Source: CAD feature listing. Evaluate the final solid. Frame: model axes, mm. A direction names the side the tool comes from. Give positions to 0.01 mm unless a question says otherwise; leave off trailing zeros. Write each loop counter-clockwise with the first axis right and the second up, starting at its lowest first coordinate (ties: lowest second). Pieces come first, ordered by that corner, then holes. Notation, with made-up numbers: (-22, 20) -> (9, 20) arc R18 cw to (9, 41) -> close; hole circle Ø3 at (46.5, 83.5). An arc over 180 degrees is marked (long way). Answer as a JSON object with one key per item and string values. Group by question number.
Item 1: First-contact query: pin 1 Ø5 at (y, z) = (-10, 3) entering from +X; pin 2 Ø4 at (y, z) = (-11, -8.5) entering from +X; pin 3 Ø1.5 at (x, z) = (16, 3.5) entering from +Y; pin 4 Ø2.5 at (x, y) = (9, -11.5) entering from -Z. Flat tips, straight axial feed; report the tip coordinate or a pass-through.
Item 2: Section query D-D on x = 19. Return the cut outline in (y, z), plus the area to 3 significant figures.
Item 3: Access query for faces 1 (the face through (14.772, -10, -5)), 2 (the face through (15.291, -15, -9)), 3 (the face through (12.576, -17.115, -3.501)). Directions: +Z, -Z, +X, -X, +Y, -Y. A direction counts if a zero-diameter tool reaches every point of the face in a straight line with its end or side. Return the directions, or none.
Item 4: Section query B-B on z = -7.75. Return the cut outline in (x, y), plus the area to 3 significant figures.
Item 5: Section query A-A on y = -9. Return the cut outline in (x, z).
Item 6: Ray query, probe 1 along X at (y, z) = (-11.45, -9); probe 2 along X at (y, z) = (-10.8, 3.5); probe 3 along Z at (x, y) = (5.75, -10.75). Return the intervals inside material, ascending. Write a range as from..to.
Item 7: Pull-direction query (X, two-part tool) for faces 4 (the face through (15.1, -10.76, -8.64)), 5 (the face through (12.253, -10, 1)), 6 (the face through (10, -10, -12.197)), 7 (the face through (14, -19, -3.2)); classes: pulls with the +X half, pulls with the -X half, needs draft (parallel to the pull), parting line crosses it, or undercut.
Item 8: Section query C-C on x = 13.75. Return the cut outline in (y, z), plus the area to 3 significant figures.
from build123d import *

# Parameters (mm, degrees)
CYLINDER054_R     = 1.75
CYLINDER054_DEPTH = 15
CYLINDER051_R     = 1.75
CYLINDER051_DEPTH = 15
EXTRUDE003_DEPTH  = 10
FILLET021_R       = 1
EXTRUDE004_DEPTH  = 5


with BuildPart() as m3holds022:
    # Cylinder054 → Cylinder054 (new body)
    with BuildSketch(Plane(origin=(6, 0.25, -9), x_dir=(1, 0, 0), z_dir=(0, -1, 0))):
        Circle(CYLINDER054_R)
    extrude(amount=CYLINDER054_DEPTH)


with BuildPart() as fusion065:
    # Cylinder051 → Cylinder051 (new body)
    with BuildSketch(Plane(origin=(14.6, 0.25, 3.5), x_dir=(1, 0, 0), z_dir=(0, -1, 0))):
        Circle(CYLINDER051_R)
    extrude(amount=CYLINDER051_DEPTH)

    # Fusion065: union m3Holds022
    add(m3holds022.part)


with BuildPart() as fillet021:
    # Sketch005 → Extrude003 (new body)
    with BuildSketch(Plane.XY):
        Polygon((57.709053, -19.346786), (57.709053, -22.346786), (65.709053, -22.346786), (65.709053, -10.346786), (62.709053, -10.346786), (62.709053, -19.346786), align=None)
    extrude(amount=EXTRUDE003_DEPTH)


with BuildPart() as fillet021_1:
    # Extrude003 placement: moved
    add(fillet021.part.moved(Location((0, 0, -14))))

    # Fillet021
    fillet021_edges = [fillet021_1.edges().sort_by_distance(p)[0] for p in [
        (57.709053, -19.346786, -9),
        (57.709053, -22.346786, -9),
        (65.709053, -22.346786, -9),
        (61.709053, -22.346786, -4),
        (65.709053, -10.346786, -9),
        (65.709053, -16.346786, -4),
        (62.709053, -10.346786, -9),
        (64.209053, -10.346786, -4),
        (62.709053, -19.346786, -9),
        (62.709053, -14.846786, -4),
        (60.209053, -19.346786, -4),
    ]]
    fillet(fillet021_edges, radius=FILLET021_R)


with BuildPart() as fillet021_2:
    # Fillet021 placement: moved
    add(fillet021_1.part.moved(Location((0, 0, 0.4))))


with BuildPart() as part_mirroring005:
    # Part__Mirroring005: instance of Fillet021
    add(fillet021_2.part.mirror(Plane(origin=(0, 0, 0), x_dir=(0, -1, 0), z_dir=(1, 0, 0))))


with BuildPart() as part_mirroring005_1:
    # Part__Mirroring005 placement: moved
    add(part_mirroring005.part.moved(Location((78, 0, 0.4))))


with BuildPart() as c4holdbottomleft:
    # Sketch006 → Extrude004 (new body)
    with BuildSketch(Plane.XZ):
        with BuildLine():
            ThreePointArc((14.771842, 0.154152), (17.827348, 3.62591), (14.461083, 6.797264))
            Line((14.461083, 6.797264), (12.252875, 6.797264))
            Line((12.252875, -5.267611), (12.252875, 6.797264))
            Line((5.422805, -5.82309), (12.252875, -5.267611))
            ThreePointArc((5.422805, -5.82309), (2.802341, -9.576998), (6.556249, -12.197462))
            Line((6.556249, -12.197462), (14.771842, -12.197462))
            Line((14.771842, -12.197462), (14.771842, 0.154152))
        make_face()
    extrude(amount=EXTRUDE004_DEPTH)


with BuildPart() as c4holdbottomleft_1:
    # Extrude004 placement: moved
    add(c4holdbottomleft.part.moved(Location((0, -8, 0))))

    # Fusion067: union Part__Mirroring005
    add(part_mirroring005_1.part)

    # Cut013: cut Fusion065
    add(fusion065.part, mode=Mode.SUBTRACT)


solid = c4holdbottomleft_1.part
Worked answers:
{
 "1": {"pin 1": "x = 17.83", "pin 2": "x = 15.29", "pin 3": "y = -8", "pin 4": "z = -12.2"},
 "2": {"outline": "(-22.35, -13.2) -> (-19.35, -13.2) -> (-19.35, -4.2) arc R1 ccw to (-20.35, -3.2) -> (-21.35, -3.2) arc R1 ccw to (-22.35, -4.2) -> close", "area": "29.6 mm^2"},
 "3": {"face 1": "+X, +Y", "face 2": "-Z, +X, +Y", "face 3": "+Z, -X, -Y"},
 "4": {"outline": "(3.01, -13) -> (4.78, -13) -> (4.78, -8) -> (3.01, -8) -> close; (7.22, -13) -> (12.29, -13) -> (12.29, -21.35) arc R1 ccw to (13.29, -22.35) -> (19.29, -22.35) arc R1 ccw to (20.29, -21.35) -> (20.29, -20.35) arc R1 ccw to (19.29, -19.35) -> (16.29, -19.35) arc R1 cw to (15.29, -18.35) -> (15.29, -11.35) arc R1 ccw to (14.77, -10.47) -> (14.77, -8) -> (7.22, -8) -> close", "area": "90.4 mm^2"},
 "5": {"outline": "(5.42, -5.82) arc R3.24 ccw to (6.56, -12.2) -> (14.77, -12.2) -> (14.77, 0.15) arc R3.33 ccw to (14.46, 6.8) -> (12.25, 6.8) -> (12.25, -5.27) -> close; hole circle Ø3.5 at (6, -9); hole circle Ø3.5 at (14.6, 3.5)"},
 "6": {"probe 1": "2.75..4.25, 7.75..15.29", "probe 2": "12.25..12.85, 16.35..17.83", "probe 3": "-12.24..-10.73, -7.27..-5.8"},
 "7": {"face 4": "pulls with the +X half", "face 5": "pulls with the -X half", "face 6": "undercut", "face 7": "needs draft"},
 "8": {"outline": "(-22.35, -13.2) -> (-10.35, -13.2) -> (-10.35, -12.2) -> (-8, -12.2) -> (-8, 1.97) -> (-13, 1.97) -> (-13, -3.2) -> (-21.35, -3.2) arc R1 ccw to (-22.35, -4.2) -> close; (-13, 5.03) -> (-8, 5.03) -> (-8, 6.8) -> (-13, 6.8) -> close", "area": "176 mm^2"}
}
